Read the model definition and answer for the solid it produces. Units are mm, in the model's axes. Face numbers are marked on the shaded views. A direction names the side the tool comes from. Give positions to 0.01 mm unless a question says otherwise; leave off trailing zeros. Order: outer loops, then holes, each group sorted by start corner. A loop starts at its lowest first (then second) coordinate and runs counter-clockwise, first axis right, second up. Notation, with made-up numbers: (59.5, 13.5) - (70.5, 13.5) arc R16 cw to (70.5, 32.5) - close; hole circle Ø6 at (41, 28). An arc over 180 degrees is marked (long way). Write each question's results on one line, items separated by ' | '.
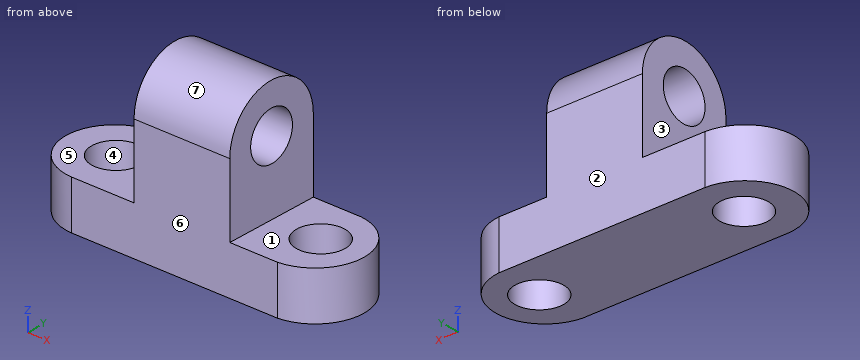
from build123d import *

# Parameters (mm, degrees)
F0_W     = 88.9
F0_H     = 63.5
F1_DEPTH = 25.4
F2_W     = 31.75
F2_H     = 50.8
F3_DEPTH = 25.4
F4_R     = 6.35
F5_DEPTH = 25.4
F6_R     = 6.35
F7_DEPTH = 25.4
F8_R     = 6.35
F9_DEPTH = 25.4


with BuildPart() as f1:
    # F0 (on Front) → F1 (new body)
    with BuildSketch(Plane.XZ):
        with Locations((1.6738499718, 31.75)):
            Rectangle(F0_W, F0_H)
    extrude(amount=F1_DEPTH)

    # F2 (on face) → F3 (cut)
    with BuildSketch(Plane.XZ.offset(25.4)):
        with Locations((-26.9011500282, 38.1)):
            Rectangle(F2_W, F2_H)
        with Locations((30.2488499718, 38.1)):
            Rectangle(F2_W, F2_H)
    extrude(amount=-F3_DEPTH, mode=Mode.SUBTRACT)

    # F4 (on face) → F5 (cut)
    with BuildSketch(Plane.YZ.offset(14.3738499718)):
        with BuildLine():
            ThreePointArc((-25.4, 31.75), (-12.7, 44.45), (0, 31.75))
            Line((0, 31.75), (0, 63.5))
            Line((0, 63.5), (-25.4, 63.5))
            Line((-25.4, 63.5), (-25.4, 31.75))
        make_face()
        with Locations((-12.7, 31.75)):
            Circle(F4_R)
    extrude(amount=-F5_DEPTH, mode=Mode.SUBTRACT)

    # F6 (on face) → F7 (cut)
    with BuildSketch(Plane.XY.offset(12.7)):
        with Locations((27.0673923413, -12.2950529623)):
            Circle(F6_R)
        with BuildLine():
            ThreePointArc((27.0673923413, 0), (38.6908388043, -12.7), (27.0673923413, -25.4))
            Line((27.0673923413, -25.4), (46.1238499718, -25.4))
            Line((46.1238499718, -25.4), (46.1238499718, 0))
            Line((46.1238499718, 0), (27.0673923413, 0))
        make_face()
    extrude(amount=-F7_DEPTH, mode=Mode.SUBTRACT)

    # F8 (on face) → F9 (cut)
    with BuildSketch(Plane.XY.offset(12.7)):
        with Locations((-26.9011500282, -12.7)):
            Circle(F8_R)
        with BuildLine():
            ThreePointArc((-27.6049521663, -25.4), (-39.9579255304, -12.7), (-27.6049521663, 0))
            Line((-27.6049521663, 0), (-42.7761500282, 0))
            Line((-42.7761500282, 0), (-42.7761500282, -25.4))
            Line((-42.7761500282, -25.4), (-27.6049521663, -25.4))
        make_face()
    extrude(amount=-F9_DEPTH, mode=Mode.SUBTRACT)


solid = f1.part
(1) Section C-C (z = 29) is taken. Give the vertices of the cut face in (x, y).
Conclusion:
outline: (-11.03, -25.4) - (14.37, -25.4) - (14.37, -18.42) - (-11.03, -18.42) - close; (-11.03, -6.98) - (14.37, -6.98) - (14.37, 0) - (-11.03, 0) - close
(2) Section A-A (y = -8) is taken. Give the vertices of the cut face in (x, z), plus the area to 3 significant figures.
Conclusion:
outline: (-39.06, 0) - (-31.17, 0) - (-31.17, 12.7) - (-39.06, 12.7) - close; (-22.63, 0) - (22.39, 0) - (22.39, 12.7) - (14.37, 12.7) - (14.37, 27.48) - (-11.03, 27.48) - (-11.03, 12.7) - (-22.63, 12.7) - close; (-11.03, 36.02) - (14.37, 36.02) - (14.37, 43.55) - (-11.03, 43.55) - close; (31.74, 0) - (37.79, 0) - (37.79, 12.7) - (31.74, 12.7) - close | area: 1,320 mm^2
(3) Consider probe 1 along X at (y, z) = (-23, 33); probe 2 along X at (y, z) = (-14.75, 10); probe 3 along Y at (x, z) = (26, 5.5). Determine where each line is inside the solid, lowest interval first. Write a range as [from, to].
Conclusion:
probe 1: [-11.03, 14.37] | probe 2: [-39.79, -32.91], [-20.89, 21.21], [32.92, 38.52] | probe 3: [-25.4, -18.55], [-6.04, 0]
(4) Each of these flat-tipped pins is pushed along its axis until it touches: pin 1 (7.5 mm diameter, centred on x = 27.07, y = -12.3, fed in from -Z); pin 2 (4 mm diameter, centred on x = 19.5, y = -22.5, fed in from +Z); pin 3 (1.5 mm diameter, centred on x = -7.5, z = 38.5, fed in from -Y); pin 4 (12.5 mm diameter, centred on y = -8, z = 27, fed in from +X). Where does it stop, or does it pass through?
Conclusion:
pin 1: through | pin 2: z = 12.7 | pin 3: y = -23.89 | pin 4: x = 14.37
(5) Section D-D (x = 23) is taken. Give the vertices of the cut face in (y, z), plus the area to 3 significant figures.
Conclusion:
outline: (-25.4, 0) - (-17.17, 0) - (-17.17, 12.7) - (-25.4, 12.7) - close; (-7.42, 0) - (0, 0) - (0, 12.7) - (-7.42, 12.7) - close | area: 199 mm^2
(6) For the marked faces 1, 2 and 3, determine the directions among +Z, -Z, +X, -X, +Y, -Y from which every point of the face is accessible in a straight line to the end or side of a thin tool.
Conclusion:
face 1: +Z, +X, +Y, -Y | face 2: +Z, -Z, +X, -X, +Y | face 3: +Z, -X, +Y, -Y
(7) Section B-B (x = 5) is taken. Give the vertices of the cut face in (y, z), plus the area to 3 significant figures.
Conclusion:
outline: (-25.4, 0) - (0, 0) - (0, 31.75) arc R12.7 ccw to (-25.4, 31.75) - close; hole circle Ø12.7 at (-12.7, 31.75) | area: 933 mm^2
(8) The mould has two halves that part along Y. Classify the marked faces 4, 5, 6 and 7: pulls with the +Y half, pulls with the -Y half, needs draft (parallel to the pull), parting line crosses it, or undercut.
Conclusion:
face 4: undercut | face 5: needs draft | face 6: pulls with the -Y half | face 7: parting line crosses it
